```python
from build123d import *

# Parameters (mm, degrees)
SKETCH_2_W                      = 15
SKETCH_2_H                      = 15
EXTRUDE_1_DEPTH                 = 7.5
SKETCH_3_W                      = 14
SKETCH_3_H                      = 4.5
CUT_EXTRUDE_1_DEPTH             = 7
SKETCH_4_R                      = 3
CUT_EXTRUDE_2_DEPTH             = 4.5
SKETCH_5_W                      = 6.5
SKETCH_5_H                      = 3.75
CUT_EXTRUDE_3_DEPTH             = 7
EXTRUDE_2_REACH                 = 20.371
SKETCH_6_R                      = 1.5
SKETCH_7_R                      = 1.25
CUT_EXTRUDE_4_DEPTH             = 19.371173071
SKETCH_8_W                      = 3
SKETCH_8_H                      = 3
EXTRUDE_3_DEPTH                 = 1
CUT_EXTRUDE_5_REACH             = 20.371
SKETCH_9_W                      = 3.5
SKETCH_9_H                      = 2
CUT_EXTRUDE_6_REACH             = 35.371
CUT_EXTRUDE_START               = -15
SKETCH_9_2_W                    = 3.5
SKETCH_9_2_H                    = 2
EXTRUDE_4_DEPTH                 = 2
EXTRUDE_4_DEPTH_BACK            = 2
CUT_EXTRUDE_7_REACH             = 14.99
CUT_EXTRUDE_7_DIRECTION_2_REACH = 14.99
FILLET_1_R                      = 0.1
FILLET_2_R                      = 0.2
SKETCH_12_R                     = 0.75
CUT_EXTRUDE_8_DEPTH             = 2


with BuildPart() as part:
    # Sketch 2 → Extrude 1 (new body)
    with BuildSketch(Plane(origin=(0, 0, 0), x_dir=(1, 0, 0), z_dir=(0, 1, 0))):
        Rectangle(SKETCH_2_W, SKETCH_2_H)
    extrude(amount=EXTRUDE_1_DEPTH)

    # Sketch 3 → Cut-Extrude 1 (cut)
    with BuildSketch(Plane(origin=(0, 7.5, 0), x_dir=(-1, 0, 0), z_dir=(0, 1, 0))):
        Rectangle(SKETCH_3_W, SKETCH_3_H)
    extrude(amount=-CUT_EXTRUDE_1_DEPTH, mode=Mode.SUBTRACT)

    # Sketch 4 → Cut-Extrude 2 (cut)
    with BuildSketch(Plane(origin=(0, 7.5, 0), x_dir=(1, 0, 0), z_dir=(0, 1, 0))):
        Circle(SKETCH_4_R)
    extrude(amount=-CUT_EXTRUDE_2_DEPTH, mode=Mode.SUBTRACT)

    # Sketch 5 → Cut-Extrude 3 (cut)
    with BuildSketch(Plane(origin=(0, 7.5, 0), x_dir=(-1, 0, 0), z_dir=(0, 1, 0))):
        with Locations((0, -5.125)):
            Rectangle(SKETCH_5_W, SKETCH_5_H)
        with Locations((0, 5.125)):
            Rectangle(SKETCH_5_W, SKETCH_5_H)
    extrude(amount=-CUT_EXTRUDE_3_DEPTH, mode=Mode.SUBTRACT)

    # Sketch 6 → Extrude 2 (add, up to next)
    with BuildSketch(Plane.XY.offset(7.5), mode=Mode.PRIVATE) as extrude_2_sk1:
        with Locations((-5, 3.75)):
            Circle(SKETCH_6_R)
    extrude_2_tool1 = extrude(extrude_2_sk1.sketch, amount=-EXTRUDE_2_REACH, mode=Mode.PRIVATE) - part.part
    # Sketch 6 → Extrude 2 (add, up to next)
    with BuildSketch(Plane.XY.offset(7.5), mode=Mode.PRIVATE) as extrude_2_sk2:
        with Locations((5, 3.75)):
            Circle(SKETCH_6_R)
    extrude_2_tool2 = extrude(extrude_2_sk2.sketch, amount=-EXTRUDE_2_REACH, mode=Mode.PRIVATE) - part.part
    add(extrude_2_tool1.solids().sort_by_distance((-5, 3.75, 7.5))[0])
    add(extrude_2_tool2.solids().sort_by_distance((5, 3.75, 7.5))[0])

    # Sketch 7 → Cut-Extrude 4 (cut, through all)
    with BuildSketch(Plane.XY.offset(7.5)):
        with Locations((-5, 3.75)):
            Circle(SKETCH_7_R)
        with Locations((5, 3.75)):
            Circle(SKETCH_7_R)
    extrude(amount=-CUT_EXTRUDE_4_DEPTH, mode=Mode.SUBTRACT)

    # Sketch 8 → Extrude 3 (add)
    with BuildSketch(Plane.XZ):
        Rectangle(SKETCH_8_W, SKETCH_8_H)
    extrude(amount=EXTRUDE_3_DEPTH)

    # Sketch 9 → Cut-Extrude 5 (cut, up to next)
    with BuildSketch(Plane.XY.offset(7.5), mode=Mode.PRIVATE) as cut_extrude_5_sk1:
        with Locations((0, 5)):
            Rectangle(SKETCH_9_W, SKETCH_9_H)
    cut_extrude_5_tool1 = extrude(cut_extrude_5_sk1.sketch, amount=-CUT_EXTRUDE_5_REACH, mode=Mode.PRIVATE) & part.part
    add(cut_extrude_5_tool1.solids().sort_by_distance((0, 5, 7.5))[0], mode=Mode.SUBTRACT)

    # Sketch 9_2 → Cut-Extrude 6 (cut, up to next)
    with BuildSketch(Plane.XY.offset(7.5).offset(CUT_EXTRUDE_START), mode=Mode.PRIVATE) as cut_extrude_6_sk1:
        with Locations((0, 5)):
            Rectangle(SKETCH_9_2_W, SKETCH_9_2_H)
    cut_extrude_6_tool1 = extrude(cut_extrude_6_sk1.sketch, amount=CUT_EXTRUDE_6_REACH, mode=Mode.PRIVATE) & part.part
    add(cut_extrude_6_tool1.solids().sort_by_distance((0, 5, -7.5))[0], mode=Mode.SUBTRACT)

    # Sketch 10 → Extrude 4 (add, two sides: drawn at the far end of the back side and taken through both)
    with BuildSketch(Plane.XY.offset(-EXTRUDE_4_DEPTH_BACK)):
        with BuildLine():
            Line((-1.95, -2.5), (1.95, -2.5))
            Line((1.95, -2.5), (1.95, -1.555590279))
            ThreePointArc((1.95, -1.555590279), (1.780042303, -1.088161527), (1.5, -0.677124344))
            Line((1.5, -0.677124344), (-1.5, -0.677124344))
            ThreePointArc((-1.5, -0.677124344), (-1.780042303, -1.088161527), (-1.95, -1.555590279))
            Line((-1.95, -1.555590279), (-1.95, -2.5))
        make_face()
    extrude(amount=EXTRUDE_4_DEPTH + EXTRUDE_4_DEPTH_BACK)

    # Sketch 11 → Cut-Extrude 7 (cut, up to next)
    with BuildSketch(Plane(origin=(0, 0, 0), x_dir=(0, 0, -1), z_dir=(1, 0, 0)), mode=Mode.PRIVATE) as cut_extrude_7_sk1:
        with BuildLine():
            Line((1.95, -2.5), (1.95, -1.555590279))
            ThreePointArc((1.95, -1.555590279), (1.780042303, -1.088161527), (1.5, -0.677124344))
            Line((1.5, -0.677124344), (2, -0.677124344))
            Line((2, -0.677124344), (2, -2.5))
            Line((2, -2.5), (1.95, -2.5))
        make_face()
    cut_extrude_7_tool1 = extrude(cut_extrude_7_sk1.sketch, amount=-CUT_EXTRUDE_7_REACH, mode=Mode.PRIVATE) & part.part
    # Sketch 11 → Cut-Extrude 7 (cut, up to next)
    with BuildSketch(Plane(origin=(0, 0, 0), x_dir=(0, 0, -1), z_dir=(1, 0, 0)), mode=Mode.PRIVATE) as cut_extrude_7_sk2:
        with BuildLine():
            Line((-1.95, -2.5), (-1.95, -1.555590279))
            ThreePointArc((-1.95, -1.555590279), (-1.780042303, -1.088161527), (-1.5, -0.677124344))
            Line((-1.5, -0.677124344), (-2, -0.677124344))
            Line((-2, -0.677124344), (-2, -2.5))
            Line((-2, -2.5), (-1.95, -2.5))
        make_face()
    cut_extrude_7_tool2 = extrude(cut_extrude_7_sk2.sketch, amount=-CUT_EXTRUDE_7_REACH, mode=Mode.PRIVATE) & part.part
    add(cut_extrude_7_tool1.solids().sort_by_distance((0, -1.175075, -1.873038))[0], mode=Mode.SUBTRACT)
    add(cut_extrude_7_tool2.solids().sort_by_distance((0, -1.175075, 1.873038))[0], mode=Mode.SUBTRACT)

    # Sketch 11 → Cut-Extrude 7 direction 2 (cut, up to next)
    with BuildSketch(Plane(origin=(0, 0, 0), x_dir=(0, 0, -1), z_dir=(1, 0, 0)), mode=Mode.PRIVATE) as cut_extrude_7_direction_2_sk1:
        with BuildLine():
            Line((1.95, -2.5), (1.95, -1.555590279))
            ThreePointArc((1.95, -1.555590279), (1.780042303, -1.088161527), (1.5, -0.677124344))
            Line((1.5, -0.677124344), (2, -0.677124344))
            Line((2, -0.677124344), (2, -2.5))
            Line((2, -2.5), (1.95, -2.5))
        make_face()
    cut_extrude_7_direction_2_tool1 = extrude(cut_extrude_7_direction_2_sk1.sketch, amount=CUT_EXTRUDE_7_DIRECTION_2_REACH, mode=Mode.PRIVATE) & part.part
    # Sketch 11 → Cut-Extrude 7 direction 2 (cut, up to next)
    with BuildSketch(Plane(origin=(0, 0, 0), x_dir=(0, 0, -1), z_dir=(1, 0, 0)), mode=Mode.PRIVATE) as cut_extrude_7_direction_2_sk2:
        with BuildLine():
            Line((-1.95, -2.5), (-1.95, -1.555590279))
            ThreePointArc((-1.95, -1.555590279), (-1.780042303, -1.088161527), (-1.5, -0.677124344))
            Line((-1.5, -0.677124344), (-2, -0.677124344))
            Line((-2, -0.677124344), (-2, -2.5))
            Line((-2, -2.5), (-1.95, -2.5))
        make_face()
    cut_extrude_7_direction_2_tool2 = extrude(cut_extrude_7_direction_2_sk2.sketch, amount=CUT_EXTRUDE_7_DIRECTION_2_REACH, mode=Mode.PRIVATE) & part.part
    add(cut_extrude_7_direction_2_tool1.solids().sort_by_distance((0, -1.175075, -1.873038))[0], mode=Mode.SUBTRACT)
    add(cut_extrude_7_direction_2_tool2.solids().sort_by_distance((0, -1.175075, 1.873038))[0], mode=Mode.SUBTRACT)

    # Fillet 1
    fillet_1_edges = [part.edges().sort_by_distance(p)[0] for p in [
        (-1.95, -2.5, 0),
        (1.95, -2.5, 0),
        (0, -2.5, -1.95),
        (0, -2.5, 1.95),
    ]]
    fillet(fillet_1_edges, radius=FILLET_1_R)

    # Fillet 2
    fillet_2_edges = [part.edges().sort_by_distance(p)[0] for p in [
        (0, 0, -7.5),
        (7.5, 0, 0),
        (0, 0, 7.5),
        (-7.5, 0, 0),
        (-7.5, 3.75, -7.5),
        (7.5, 3.75, -7.5),
        (7.5, 3.75, 7.5),
        (-7.5, 3.75, 7.5),
    ]]
    fillet(fillet_2_edges, radius=FILLET_2_R)

    # Sketch 12 → Cut-Extrude 8 (cut)
    with BuildSketch(Plane(origin=(0, 7.5, 0), x_dir=(-1, 0, 0), z_dir=(0, 1, 0))):
        with Locations(Location((6.5, -6.5, 0), (0, 0, 90))):
            Circle(SKETCH_12_R)
        with Locations(Location((-6.5, 6.5, 0), (0, 0, 90))):
            Circle(SKETCH_12_R)
        with Locations(Location((6.5, 6.5, 0), (0, 0, 90))):
            Circle(SKETCH_12_R)
        with Locations(Location((-6.5, -6.5, 0), (0, 0, 90))):
            Circle(SKETCH_12_R)
    extrude(amount=-CUT_EXTRUDE_8_DEPTH, mode=Mode.SUBTRACT)


solid = part.part
```
Geometry check sheet. Reference: the model listing, model coordinates, mm. A direction names the side the tool comes from. Round coordinates to 2 decimals unless told otherwise and drop trailing zeros. Order: outer loops, then holes, each group sorted by start corner. A loop starts at its lowest first (then second) coordinate and runs counter-clockwise, first axis right, second up. Notation, with made-up numbers: (-14.75, 56.25) -> (6.25, 56.25) arc R20 cw to (6.25, 90.25) -> close; hole circle Ø3 at (43, -25). An arc over 180 degrees is marked (long way). Return JSON: item names as keys, results as strings. Group by question number.
Q1. Material ranges on probe 1 along Z at (x, y) = (-2.5, 2.5); probe 2 along X at (y, z) = (7.05, -6.5), recorded low to high. Write a range as from..to.
Q2. Section check A-A, the plane x = -5. Record the boundary of the cut face in (y, z).
Q3. Release check for a two-part mould opening along Z. For faces 1 (the cylindrical face through (-6.47, 6.51, -7.25)), 2 (the flat face through (-7.5, 4, 0)), 3 (the flat face through (-0.1, 3.8, -7.5)) record: released by +Z, released by -Z, zero draft, split by the parting line, or undercut.
Q4. Tool access check on faces 4 (the flat face through (0, 0.5, 5)), 5 (the cylindrical face through (6.386, 3.175, 0.031)), 6 (the cylindrical face through (1.78, -1.09, -0.03)), 7 (the flat face through (0, -2, 1.95)). Record the directions out of +Z, -Z, +X, -X, +Y, -Y that give a thin tool (end or side, any length) a straight path to the whole face; none if there is none.
Q5. Section check C-C, the plane z = -5.5. Record the boundary of the cut face in (x, y), plus the area to 3 significant figures.
Q6. Section check D-D, the plane x = 0. Count the separate pieces of the cut face and the enclosed holes in it, plus the area to 3 significant figures.
Q7. Section check B-B, the plane y = 6.75. Record the boundary of the cut face in (x, z).
Q8. Gauge pin test, flat ends, axial feed: pin 1 (2 mm diameter, centred on x = 6.5, z = 6.5, fed in from -Y); pin 2 (0.7 mm diameter, centred on x = -0.5, y = -2, fed in from -Z); pin 3 (0.9 mm diameter, centred on x = 0.5, y = -2, fed in from +Z). Record the tip position at first contact, or that the pin passes through.
Numbers:
{
 "1": {"probe 1": "-7.5..-7, -3.25..-2.25, 2.25..3.25, 7..7.5", "probe 2": "-7.5..-7.25, -5.75..-3.25, 3.25..5.75, 7.25..7.5"},
 "2": {"outline": "(0, -7.3) arc R0.2 ccw to (0.2, -7.5) -> (2.5, -7.5) -> (2.5, 7.5) -> (0.2, 7.5) arc R0.2 ccw to (0, 7.3) -> close; (5, -7.5) -> (7.5, -7.5) -> (7.5, -2.25) -> (5.25, -2.25) -> (5.25, 2.25) -> (7.5, 2.25) -> (7.5, 7.5) -> (5, 7.5) -> close; hole (0.5, -2.25) -> (2.25, -2.25) -> (2.25, 2.25) -> (0.5, 2.25) -> close"},
 "3": {"face 1": "undercut", "face 2": "zero draft", "face 3": "released by -Z"},
 "4": {"face 4": "+Y", "face 5": "none", "face 6": "+Z, -Z, +X", "face 7": "+Z, +X, -X, -Y"},
 "5": {"outline": "(-7.5, 0.2) arc R0.2 ccw to (-7.3, 0) -> (7.3, 0) arc R0.2 ccw to (7.5, 0.2) -> (7.5, 7.5) -> (3.25, 7.5) -> (3.25, 0.5) -> (-3.25, 0.5) -> (-3.25, 7.5) -> (-7.5, 7.5) -> close; hole circle Ø2.5 at (-5, 3.75); hole circle Ø2.5 at (5, 3.75)", "area": "57.2 mm^2"},
 "6": {"separate pieces": "3", "enclosed holes": "0", "area": "28.6 mm^2"},
 "7": {"outline": "(-7.5, -7.3) arc R0.2 ccw to (-7.3, -7.5) -> (7.3, -7.5) arc R0.2 ccw to (7.5, -7.3) -> (7.5, 7.3) arc R0.2 ccw to (7.3, 7.5) -> (-7.3, 7.5) arc R0.2 ccw to (-7.5, 7.3) -> close; hole circle Ø1.5 at (-6.5, -6.5); hole circle Ø1.5 at (-6.5, 6.5); hole (-7, -2.25) -> (-1.98, -2.25) arc R3 ccw to (1.98, -2.25) -> (7, -2.25) -> (7, 2.25) -> (1.98, 2.25) arc R3 ccw to (-1.98, 2.25) -> (-7, 2.25) -> close; hole (-3.25, -7) -> (3.25, -7) -> (3.25, -3.25) -> (-3.25, -3.25) -> close; hole (-3.25, 3.25) -> (3.25, 3.25) -> (3.25, 7) -> (-3.25, 7) -> close; hole circle Ø1.5 at (6.5, -6.5); hole circle Ø1.5 at (6.5, 6.5)"},
 "8": {"pin 1": "y = 0", "pin 2": "z = -1.95", "pin 3": "z = 1.95"}
}
